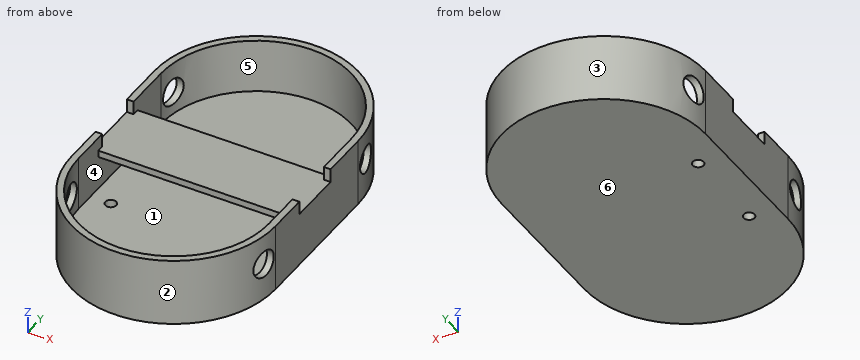
from build123d import *

# Parameters (mm, degrees)
CYLINDER049_R           = 0.8
CYLINDER049_DEPTH       = 10
CYLINDER048_R           = 0.8
CYLINDER048_DEPTH       = 10
BOX013_W                = 28
BOX013_H                = 10
BOX013_DEPTH            = 2
BOX011_W                = 28
BOX011_H                = 10
BOX011_DEPTH            = 3
CYLINDER029_R           = 2
CYLINDER029_DEPTH       = 10
CYLINDER029_PITCH_ANGLE = 90
CYLINDER031_R           = 2
CYLINDER031_DEPTH       = 10
CYLINDER031_PITCH_ANGLE = 90
CYLINDER030_R           = 2
CYLINDER030_DEPTH       = 10
CYLINDER030_PITCH_ANGLE = 90
CYLINDER028_R           = 2
CYLINDER028_DEPTH       = 10
CYLINDER028_PITCH_ANGLE = 90
BOX012_W                = 33
BOX012_H                = 8
BOX012_DEPTH            = 2
CYLINDER002_W           = 14
CYLINDER002_H           = 8
CYLINDER002_ANGLE       = 180
CYLINDER001_W           = 15
CYLINDER001_H           = 10
CYLINDER001_ANGLE       = 180
CYLINDER003_W           = 14
CYLINDER003_H           = 8
CYLINDER003_ANGLE       = 180
CYLINDER_W              = 15
CYLINDER_H              = 10
CYLINDER_ANGLE          = 180
BOX001_W                = 28
BOX001_H                = 21
BOX001_DEPTH            = 8
BOX_W                   = 30
BOX_H                   = 21
BOX_DEPTH               = 10
FUSION_PLACEMENT_ANGLE  = 180


with BuildPart() as cilindro049:
    # Cylinder049 → Cylinder049 (new body)
    with BuildSketch(Plane(origin=(-10, -18, -15), x_dir=(1, 0, 0), z_dir=(0, 0, 1))):
        Circle(CYLINDER049_R)
    extrude(amount=CYLINDER049_DEPTH)


with BuildPart() as cilindro048:
    # Cylinder048 → Cylinder048 (new body)
    with BuildSketch(Plane(origin=(-10, -5, -15), x_dir=(1, 0, 0), z_dir=(0, 0, 1))):
        Circle(CYLINDER048_R)
    extrude(amount=CYLINDER048_DEPTH)


with BuildPart() as cubo013:
    # Box013 → Box013 (new body)
    with BuildSketch(Plane(origin=(-27, 54, 42), x_dir=(1, 0, 0), z_dir=(0, 0, 1))):
        with Locations((14, 5)):
            Rectangle(BOX013_W, BOX013_H)
    extrude(amount=BOX013_DEPTH)


with BuildPart() as cut004:
    # Box011 → Box011 (new body)
    with BuildSketch(Plane(origin=(-27, 54, 41), x_dir=(1, 0, 0), z_dir=(0, 0, 1))):
        with Locations((14, 5)):
            Rectangle(BOX011_W, BOX011_H)
    extrude(amount=BOX011_DEPTH)

    # Cut004: cut Cubo013
    add(cubo013.part, mode=Mode.SUBTRACT)


with BuildPart() as cilindro029:
    # Cylinder029 → Cylinder029 (new body)
    with BuildSketch(Plane.XY):
        Circle(CYLINDER029_R)
    extrude(amount=CYLINDER029_DEPTH)


with BuildPart() as cilindro029_1:
    # Cylinder029 pitch: moved
    add(cilindro029.part.rotate(Axis((0, 0, 0), (0, 1, 0)), CYLINDER029_PITCH_ANGLE))


with BuildPart() as cilindro029_2:
    # Cylinder029 placement: moved
    add(cilindro029_1.part.moved(Location((-29, 46.5, 39.5))))


with BuildPart() as cilindro031:
    # Cylinder031 → Cylinder031 (new body)
    with BuildSketch(Plane.XY):
        Circle(CYLINDER031_R)
    extrude(amount=CYLINDER031_DEPTH)


with BuildPart() as cilindro031_1:
    # Cylinder031 pitch: moved
    add(cilindro031.part.rotate(Axis((0, 0, 0), (0, 1, 0)), CYLINDER031_PITCH_ANGLE))


with BuildPart() as cilindro031_2:
    # Cylinder031 placement: moved
    add(cilindro031_1.part.moved(Location((-5, 72.5, 39.5))))


with BuildPart() as cilindro030:
    # Cylinder030 → Cylinder030 (new body)
    with BuildSketch(Plane.XY):
        Circle(CYLINDER030_R)
    extrude(amount=CYLINDER030_DEPTH)


with BuildPart() as cilindro030_1:
    # Cylinder030 pitch: moved
    add(cilindro030.part.rotate(Axis((0, 0, 0), (0, 1, 0)), CYLINDER030_PITCH_ANGLE))


with BuildPart() as cilindro030_2:
    # Cylinder030 placement: moved
    add(cilindro030_1.part.moved(Location((-5, 46.5, 39.5))))


with BuildPart() as cilindro028:
    # Cylinder028 → Cylinder028 (new body)
    with BuildSketch(Plane.XY):
        Circle(CYLINDER028_R)
    extrude(amount=CYLINDER028_DEPTH)


with BuildPart() as cilindro028_1:
    # Cylinder028 pitch: moved
    add(cilindro028.part.rotate(Axis((0, 0, 0), (0, 1, 0)), CYLINDER028_PITCH_ANGLE))


with BuildPart() as cilindro028_2:
    # Cylinder028 placement: moved
    add(cilindro028_1.part.moved(Location((-29, 72.5, 39.5))))


with BuildPart() as cubo012:
    # Box012 → Box012 (new body)
    with BuildSketch(Plane(origin=(-30, 55, 42), x_dir=(1, 0, 0), z_dir=(0, 0, 1))):
        with Locations((16.5, 4)):
            Rectangle(BOX012_W, BOX012_H)
    extrude(amount=BOX012_DEPTH)


with BuildPart() as cilindro002:
    # Cylinder002 → Cylinder002 (revolve)
    with BuildSketch(Plane(origin=(16, 49, -36), x_dir=(1, 0, 0), z_dir=(0, 1, 0))):
        with Locations((7, 4)):
            Rectangle(CYLINDER002_W, CYLINDER002_H)
    revolve(axis=Axis((16, 49, -36), (0, 0, -1)), revolution_arc=CYLINDER002_ANGLE)


with BuildPart() as cut001:
    # Cylinder001 → Cylinder001 (revolve)
    with BuildSketch(Plane(origin=(16, 49, -34), x_dir=(1, 0, 0), z_dir=(0, 1, 0))):
        with Locations((7.5, 5)):
            Rectangle(CYLINDER001_W, CYLINDER001_H)
    revolve(axis=Axis((16, 49, -34), (0, 0, -1)), revolution_arc=CYLINDER001_ANGLE)

    # Cut001: cut Cilindro002
    add(cilindro002.part, mode=Mode.SUBTRACT)


with BuildPart() as cut001_1:
    # Cut001 placement: moved
    add(cut001.part.moved(Location((-3, 0, 0))))


with BuildPart() as cilindro003:
    # Cylinder003 → Cylinder003 (revolve)
    with BuildSketch(Plane(origin=(13, 70, -36), x_dir=(-1, 0, 0), z_dir=(0, -1, 0))):
        with Locations((7, 4)):
            Rectangle(CYLINDER003_W, CYLINDER003_H)
    revolve(axis=Axis((13, 70, -36), (0, 0, -1)), revolution_arc=CYLINDER003_ANGLE)


with BuildPart() as cut002:
    # Cylinder → Cylinder (revolve)
    with BuildSketch(Plane(origin=(13, 70, -34), x_dir=(-1, 0, 0), z_dir=(0, -1, 0))):
        with Locations((7.5, 5)):
            Rectangle(CYLINDER_W, CYLINDER_H)
    revolve(axis=Axis((13, 70, -34), (0, 0, -1)), revolution_arc=CYLINDER_ANGLE)

    # Cut002: cut Cilindro003
    add(cilindro003.part, mode=Mode.SUBTRACT)


with BuildPart() as cubo001:
    # Box001 → Box001 (new body)
    with BuildSketch(Plane(origin=(-1, 49, -44), x_dir=(1, 0, 0), z_dir=(0, 0, 1))):
        with Locations((14, 10.5)):
            Rectangle(BOX001_W, BOX001_H)
    extrude(amount=BOX001_DEPTH)


with BuildPart() as cut068:
    # Box → Box (new body)
    with BuildSketch(Plane(origin=(-2, 49, -44), x_dir=(1, 0, 0), z_dir=(0, 0, 1))):
        with Locations((15, 10.5)):
            Rectangle(BOX_W, BOX_H)
    extrude(amount=BOX_DEPTH)

    # Cut: cut Cubo001
    add(cubo001.part, mode=Mode.SUBTRACT)

    # Fusion: union Cut001, Cut002
    add(cut001_1.part)
    add(cut002.part)


with BuildPart() as cut068_1:
    # Fusion placement: moved
    add(cut068.part.rotate(Axis((0, 0, 0), (0, 1, 0)), FUSION_PLACEMENT_ANGLE))

    # Cut003: cut Cubo012
    add(cubo012.part, mode=Mode.SUBTRACT)

    # Cut040: cut Cilindro028
    add(cilindro028_2.part, mode=Mode.SUBTRACT)

    # Cut041: cut Cilindro030
    add(cilindro030_2.part, mode=Mode.SUBTRACT)

    # Cut042: cut Cilindro031
    add(cilindro031_2.part, mode=Mode.SUBTRACT)

    # Cut043: cut Cilindro029
    add(cilindro029_2.part, mode=Mode.SUBTRACT)

    # Fusion002019: union Cut004
    add(cut004.part)


with BuildPart() as cut068_2:
    # Fusion002019 placement: moved
    add(cut068_1.part.moved(Location((14, -70, -44))))

    # Cut067: cut Cilindro048
    add(cilindro048.part, mode=Mode.SUBTRACT)

    # Cut068: cut Cilindro049
    add(cilindro049.part, mode=Mode.SUBTRACT)


solid = cut068_2.part
Geometry: final body of the model. Coordinates: model frame, mm. Face numbers are marked on the shaded views. A direction names the side the tool comes from. Give positions to 0.01 mm unless a question says otherwise; leave off trailing zeros. Write each loop counter-clockwise with the first axis right and the second up, starting at its lowest first coordinate (ties: lowest second). Pieces come first, ordered by that corner, then holes. Notation, with made-up numbers: M 32,32 L 62,32 A27 ccw 62,56 Z; hole C 45.5,57 d3. An arc over 180 degrees is marked long. Answer in a Markdown table with one row per item. Add a question column.
(1) Mould query, pull axis X, two halves, no side actions, for the marked faces 3, 4, 5 and 6. Classes: +X half, -X half, draft (parallel to the pull), parting line (faces both ways), or undercut.
(2) Section B-B on y = -18. Return loops of the section in (x, z).
(3) Section D-D on y = -23.5. Return loops of the section in (x, z).
(4) First-contact query: pin 1 (3 mm diameter, centred on y = -23.5, z = -4.5, fed in from -X); pin 2 (8 mm diameter, centred on x = 8, y = -9, fed in from +Z); pin 3 (6 mm diameter, centred on x = 13, z = -3, fed in from -Y); pin 4 (0.5 mm diameter, centred on x = 5.5, z = -2.5, fed in from +Y). Flat tips, straight axial feed; report the tip coordinate or a pass-through.
(5) Section A-A on z = -7. Return loops of the section in (x, y), and give its area (3 significant figures).
(6) Ray query, line 1 (Z direction, x = 0, y = -8.5); line 2 (Z direction, x = 15.35, y = -23.5); line 3 (Y direction, x = -10, z = -9.05). Return the intervals inside material, ascending.
(7) Section C-C on x = 1. Return loops of the section in (y, z), and give its area (3 significant figures).
(8) Reachability of the marked faces 1 and 2 from +Z, -Z, +X, -X, +Y, -Y: full face, straight path, thin tool, end or side. Return the list, or none.
Result set:
| question | item | result |
|---|---|---|
| 1 | face 3 | parting line |
| 1 | face 4 | undercut |
| 1 | face 5 | undercut |
| 1 | face 6 | draft |
| 2 | outline | M -14,-10 L -10.8,-10 L -10.8,-8 L -13,-8 L -13,0 L -14,0 Z; M -9.2,-10 L 16,-10 L 16,0 L 15,0 L 15,-8 L -9.2,-8 Z |
| 3 | outline | M -13.79,-10 L 15.79,-10 L 15.79,-6.5 L 14.77,-6.5 L 14.77,-8 L -12.77,-8 L -12.77,-6.5 L -13.79,-6.5 Z; M -13.79,-2.5 L -12.77,-2.5 L -12.77,0 L -13.79,0 Z; M 14.77,-2.5 L 15.79,-2.5 L 15.79,0 L 14.77,0 Z |
| 4 | pin 1 | passes through |
| 4 | pin 2 | stops at z = -2 |
| 4 | pin 3 | stops at y = -33 |
| 4 | pin 4 | stops at y = 14.39 |
| 5 | outline | M -14,-21 A15 ccw 16,-21 L 16,0 A15 ccw -14,0 Z; hole M -13,-21 A14 ccw 15,-21 L 15,0 A14 ccw -13,0 Z |
| 5 | area | 133 mm^2 |
| 6 | line 1 | z = -10 to -8, -3 to -2 |
| 6 | line 2 | z = -10 to -6.5, -2.5 to 0 |
| 6 | line 3 | y = -31.2 to -18.8, -17.2 to -5.8, -4.2 to 10.2 |
| 7 | outline | M -36,-10 L 15,-10 L 15,0 L 14,0 L 14,-8 L -35,-8 L -35,0 L -36,0 Z; M -16,-3 L -6,-3 L -6,-2 L -16,-2 Z |
| 7 | area | 128 mm^2 |
| 8 | face 1 | none |
| 8 | face 2 | +Z, -Z, -Y |
